from build123d import *

# Parameters (mm, degrees)
F0_R     = 4
F1_DEPTH = 2


with BuildPart() as f1:
    # F0 (on Top) → F1 (new body)
    with BuildSketch(Plane.XY):
        with BuildLine():
            Line((-15.434873, 25.724788), (-58.309519, 0))
            Line((-58.309519, 0), (-15.434873, -25.724788))
            ThreePointArc((-15.434873, -25.724788), (30, 0), (-15.434873, 25.724788))
        make_face()
        with Locations((15, -15)):
            Circle(F0_R, mode=Mode.SUBTRACT)
        with Locations((-25, 0)):
            Circle(F0_R, mode=Mode.SUBTRACT)
        with Locations((15, 15)):
            Circle(F0_R, mode=Mode.SUBTRACT)
    extrude(amount=F1_DEPTH)


solid = f1.part
Source: CAD feature listing. Evaluate the final solid. Frame: model axes, mm. Give positions to 0.01 mm unless a question says otherwise; leave off trailing zeros. Write each loop counter-clockwise with the first axis right and the second up, starting at its lowest first coordinate (ties: lowest second). Pieces come first, ordered by that corner, then holes. Notation, with made-up numbers: (-2, 18.25) - (2, 18.25) arc R31 ccw to (2, 49.25) - close; hole circle Ø9 at (77.25, 72.5). An arc over 180 degrees is marked (long way). Write item = value, one per line. Start each with the question number.
Q1. Material intervals for probe 1 along Y at (x, z) = (12.5, 0.15); probe 2 along Y at (x, z) = (15, 0.6); probe 3 along Y at (x, z) = (-25, 0.6), sorted ascending.
Q2. Pin query (flat end, axial travel): pin 1 Ø1 at (y, z) = (23, 0.5) entering from -X; pin 2 Ø9 at (x, y) = (-25, 0) entering from +Z. Return the tip coordinate at first contact, or that it passes through.
Q3. Cut plane C-C, the plane z = 0.35. Return loops of the section in (x, y).
Q4. Draft query along X for faces 1 (the cylindrical face through (11, -15, 1)), 2 (the cylindrical face through (29.987, -0.887, 0.986)), 3 (the flat face through (-36.572, 13.042, 0.986)). Return one class per face: +X half, -X half, draft (parallel to the pull), parting line (faces both ways), or undercut.
Q5. Cut plane B-B, the plane x = 15. Return loops of the section in (y, z).
Q6. Cut plane D-D, the plane x = -25. Return loops of the section in (y, z).
Q7. Cut plane A-A, the plane y = -15. Return loops of the section in (x, z), then the cut area to 3 significant figures.
Computed values:
q1.probe_1 = -27.27 to -18.12, -11.88 to 11.88, 18.12 to 27.27
q1.probe_2 = -25.98 to -19, -11 to 11, 19 to 25.98
q1.probe_3 = -19.99 to -4, 4 to 19.99
q2.pin_1 = -20.81
q2.pin_2 = 2
q3.outline = (-58.31, 0) - (-15.43, -25.72) arc R30 ccw (long way) to (-15.43, 25.72) - close; hole circle Ø8 at (-25, 0); hole circle Ø8 at (15, -15); hole circle Ø8 at (15, 15)
q4.face_1 = undercut
q4.face_2 = parting line
q4.face_3 = -X half
q5.outline = (-25.98, 0) - (-19, 0) - (-19, 2) - (-25.98, 2) - close; (-11, 0) - (11, 0) - (11, 2) - (-11, 2) - close; (19, 0) - (25.98, 0) - (25.98, 2) - (19, 2) - close
q6.outline = (-19.99, 0) - (-4, 0) - (-4, 2) - (-19.99, 2) - close; (4, 0) - (19.99, 0) - (19.99, 2) - (4, 2) - close
q7.outline = (-33.31, 0) - (11, 0) - (11, 2) - (-33.31, 2) - close; (19, 0) - (25.98, 0) - (25.98, 2) - (19, 2) - close
q7.area = 103 mm²
